Study the drawing (mm; zero at the part's minimum x, y, z) and answer. Give positions to 0.01 mm unless a question says otherwise; leave off trailing zeros. Loops run counter-clockwise (first coordinate to the right, second up) from the corner with the lowest first, then second, coordinate; pieces in that order, holes last. Notation, with made-up numbers: M -29.5,43.25 L 28.5,43.25 A27 ccw 28.5,69.25 Z; hole C 30.25,1 d1. An arc over 180 degrees is marked long. Use one line per item in the form item = value. Start each with the question number.
1. This flat-tipped pin is pushed along its axis until it touches: pin 1 Ø1.5 at (y, z) = (26.5, 2.5) entering from -X. Where does it stop, or does it pass through?
2. The part is cut by section B-B (z = 5.25). Write down the section's boundary in (x, y), and give its area (3 significant figures).
3. The part is cut by section D-D (y = 49). Write down the section's boundary in (x, z), and give its area (4 significant figures).
4. Straight lines are drawn through the part: line 1 (X direction, y = 41, z = 1.5); line 2 (X direction, y = 54, z = 2). For each, find the intervals that lie inside material, in ascending order. Write a range as from..to.
5. The part is cut by section A-A (y = 41). Write down the section's boundary in (x, z).
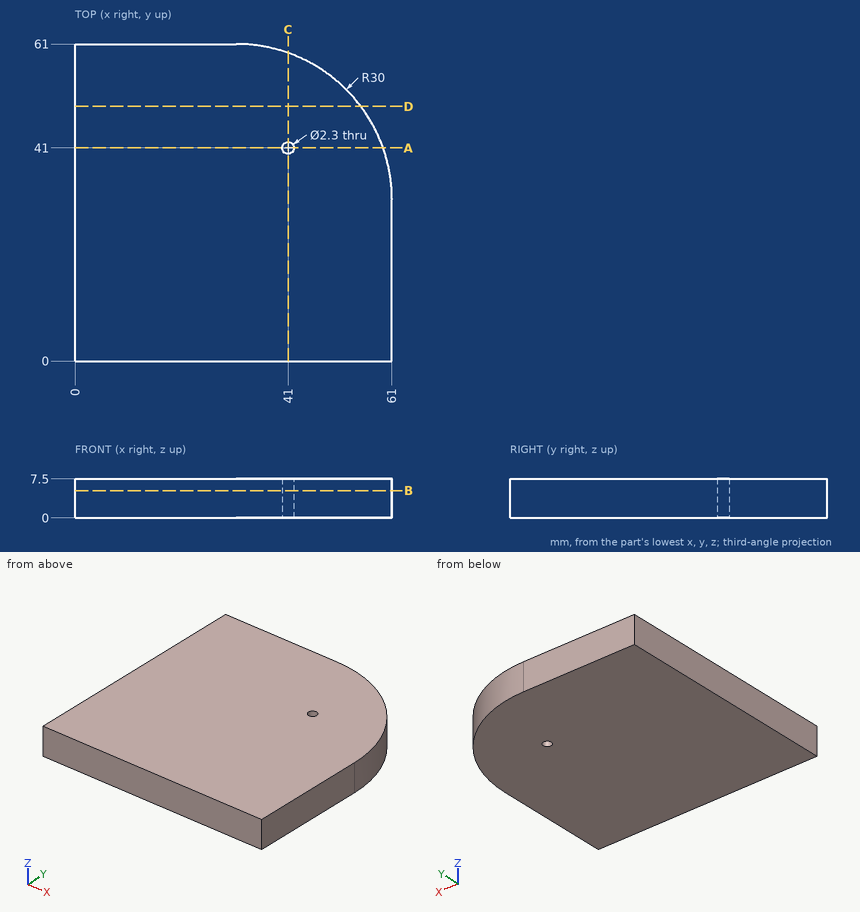
Derived:
q1.pin_1 = 0
q2.outline = M 0,0 L 61,0 L 61,31 A30 ccw 31,61 L 0,61 Z; hole C 41,41 d2.3
q2.area = 3,520 mm2
q3.outline = M 0,0 L 55,0 L 55,7.5 L 0,7.5 Z
q3.area = 412.5 mm2
q4.line_1 = 0..39.85, 42.15..59.28
q4.line_2 = 0..50.26
q5.outline = M 0,0 L 39.85,0 L 39.85,7.5 L 0,7.5 Z; M 42.15,0 L 59.28,0 L 59.28,7.5 L 42.15,7.5 Z
